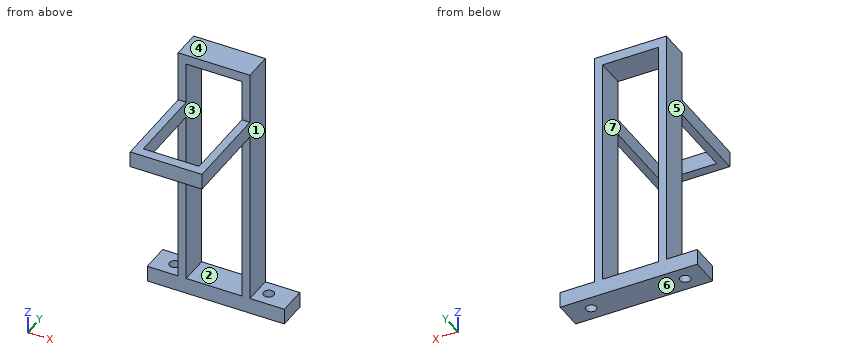
Autodesk Inventor part; units mm, degrees
ref_plane "YZ Plane" through (0, 0, 0) normal (1, 0, 0) x (0, 1, 0)
ref_plane "XZ Plane" through (0, 0, 0) normal (0, 1, 0) x (-1, 0, 0)
ref_plane "XY Plane" through (0, 0, 0) normal (0, 0, 1) x (1, 0, 0)
sketch "Sketch1" plane through (0, 0, 0) normal (0, 0, 1) x (1, 0, 0)
  line L0 (0, 0) -> (43, 0)
  line L1 (43, 0) -> (43, 9)
  line L2 (43, 9) -> (0, 9)
  line L3 (0, 9) -> (0, 0)
  dimension "d0" = 43
  dimension "d1" = 9
extrude "Extrusion1" add sketch "Sketch1" along normal blind 5
sketch "Sketch2" plane through (0, 0, 5) normal (0, 0, 1) x (1, 0, 0)
  line L0 (43, 0) -> (43, 9)
  line L1 (43, 9) -> (0, 9)
  point P0 (0, 0)
  point P1 (35.7, 4.5)
  point P2 (6.2, 4.5)
  dimension "d11" = 7.3
  dimension "d12" = 29.5
  dimension "d13" = 4.5
  dimension "d14" = 4.5
hole "Hole1" at (35.7, 4.5, 5) at (6.2, 4.5, 5) direction (0, 0, -1) diameter 3.3 end through all
sketch "Sketch3" plane through (0, 0, 5) normal (0, 0, 1) x (1, 0, 0)
  line L0 (0, 0) -> (43, 0)
  line L1 (43, 9) -> (0, 9)
  line L2 (9.7, 0) -> (12.2, 0)
  line L3 (12.2, 0) -> (12.2, 9)
  line L4 (12.2, 9) -> (9.7, 9)
  line L5 (9.7, 9) -> (9.7, 0)
  line L6 (29.7, 9) -> (32.2, 9)
  line L7 (32.2, 9) -> (32.2, 0)
  line L8 (32.2, 0) -> (29.7, 0)
  line L9 (29.7, 0) -> (29.7, 9)
  circle A0 centre (35.7, 4.5) radius 1.65
  point P0 (29.7, 4.5)
  point P1 (12.2, 4.5)
  point P2 (32.2, 4.5)
  point P3 (29.7, 9)
  point P4 (29.7, 0)
  point P5 (32.2, 0)
  point P6 (32.2, 9)
  point P7 (12.2, 0)
  dimension "d15" = 2.5
  dimension "d16" = 2.5
  dimension "d17" = 17.5
  dimension "d18" = 3.5
extrude "Extrusion2" add sketch "Sketch3" along normal blind 76 contours L5 L1 L3 L0 | L9 L1 L7 L0
sketch "Sketch4" plane through (0, 0, 81) normal (0, 0, 1) x (1, 0, 0)
  line L0 (12.2, 9) -> (9.7, 9)
  line L1 (32.2, 0) -> (9.7, 0)
  line L2 (9.7, 0) -> (9.7, 9)
  line L3 (9.7, 9) -> (32.2, 9)
  line L4 (32.2, 9) -> (32.2, 0)
  point P0 (0, 0)
extrude "Extrusion3" add sketch "Sketch4" against normal blind 3
sketch "Sketch7" plane through (0, 0, 0) normal (0, -1, 0) x (1, 0, 0)
  line L0 (9.7, 60) -> (9.7, 65)
  line L1 (9.7, 65) -> (12.2, 65)
  line L2 (12.2, 65) -> (12.2, 60)
  line L3 (12.2, 60) -> (9.7, 60)
  line L4 (9.7, 60) -> (9.7, 65)
  line L5 (32.2, 65) -> (29.7, 65)
  line L6 (29.7, 65) -> (32.2, 65)
  line L7 (32.2, 65) -> (32.2, 60)
  line L8 (32.2, 60) -> (29.7, 60)
  line L9 (29.7, 60) -> (29.7, 65)
  point P0 (0, 0)
  dimension "d31" = 2.5
  dimension "d32" = 5
extrude "Extrusion6" add sketch "Sketch7" along normal blind 28
sketch "Sketch8" plane through (29.7, 0, 5) normal (-1, 0, 0) x (0, 0, 1)
  line L0 (60, 0) -> (60, -28)
  line L1 (60, -28) -> (55, -28)
  line L2 (55, -28) -> (55, -25)
  line L3 (55, -25) -> (60, -25)
  line L4 (60, -25) -> (60, -28)
  point P0 (-5, 0)
  dimension "d35" = 5
  dimension "d36" = 3
extrude "Extrusion7" add sketch "Sketch8" along normal blind 18
properties part number "Batteryholder1"
Geometry check sheet. Reference: the model listing, model coordinates, mm. Face numbers are marked on the shaded views. A direction names the side the tool comes from. Coordinates: 2 decimals unless noted, no trailing zeros. Order: outer loops, then holes, each group sorted by start corner. A loop starts at its lowest first (then second) coordinate and runs counter-clockwise, first axis right, second up. Notation, with made-up numbers: M 37.5,3.5 L 94.5,3.5 A25 ccw 94.5,38.5 Z; hole C -23.75,17 d8. An arc over 180 degrees is marked long. One line per question, with ' | ' between items. Start each with the question number.
Item 1: Gauge pin test, flat ends, axial feed: pin 1 (6 mm diameter, centred on x = 13.5, y = -6, fed in from -Z); pin 2 (5.5 mm diameter, centred on x = 23.5, z = 62.5, fed in from +Y); pin 3 (4.5 mm diameter, centred on x = 6.5, y = 5.5, fed in from +Z). Record the tip position at first contact, or that the pin passes through.
Item 2: Cross-section at C-C on x = 6.2. Enter the section's corners in (y, z).
Item 3: Cross-section at B-B on z = 69. Enter the section's corners in (x, y), then the cut area to 3 significant figures.
Item 4: Material ranges on L1, parallel to X at y = 4.5, z = 2.7; L2, parallel to Y at x = 6, z = 1; L3, parallel to X at y = 1.5, z = 14.5, recorded low to high. Write a range as [from, to].
Item 5: Set-up check for the marked faces 1, 2, 3 and 4: record each of +Z, -Z, +X, -X, +Y, -Y from which the full face is reachable in a straight line by a thin tool's end or side.
Item 6: Draft check along Z on the marked faces 5, 6 and 7. Enter one of: pulls with the +Z half, pulls with the -Z half, needs draft (parallel to the pull), parting line crosses it, or undercut.
Item 7: Cross-section at D-D on x = 19. Enter the section's corners in (y, z).
Item 8: Cross-section at A-A on y = 4.5. Enter the section's corners in (x, z).
Findings:
1) pin 1: stops at z = 60 | pin 2: stops at y = -25 | pin 3: stops at z = 5
2) outline: M 0,0 L 2.85,0 L 2.85,5 L 0,5 Z; M 6.15,0 L 9,0 L 9,5 L 6.15,5 Z
3) outline: M 9.7,0 L 12.2,0 L 12.2,9 L 9.7,9 Z; M 29.7,0 L 32.2,0 L 32.2,9 L 29.7,9 Z | area: 45.0 mm²
4) L1: x = [0, 4.55], [7.85, 34.05], [37.35, 43] | L2: y = [0, 2.86], [6.14, 9] | L3: x = [9.7, 12.2], [29.7, 32.2]
5) face 1: +Z, +X, +Y, -Y | face 2: +Y, -Y | face 3: +Y | face 4: +Z, +X, -X, +Y, -Y
6) face 5: needs draft | face 6: pulls with the -Z half | face 7: undercut
7) outline: M -28,60 L -25,60 L -25,65 L -28,65 Z; M 0,0 L 9,0 L 9,5 L 0,5 Z; M 0,78 L 9,78 L 9,81 L 0,81 Z
8) outline: M 0,0 L 4.55,0 L 4.55,5 L 0,5 Z; M 7.85,0 L 34.05,0 L 34.05,5 L 32.2,5 L 32.2,81 L 9.7,81 L 9.7,5 L 7.85,5 Z; M 37.35,0 L 43,0 L 43,5 L 37.35,5 Z; hole M 12.2,5 L 29.7,5 L 29.7,78 L 12.2,78 Z
